Build history of the part. All positions in model axes, mm. A direction names the side the tool comes from. Give positions to 0.01 mm unless a question says otherwise; leave off trailing zeros. Loops run counter-clockwise (first coordinate to the right, second up) from the corner with the lowest first, then second, coordinate; pieces in that order, holes last.
1) Two-plate mould, pull along Z, no slides. Class faces 6 (the flat face through (28, 1, 23)), 7 (the flat face through (-22.4, 22, 12.4)), 8 (the flat face through (0, 12, 12)), 9 (the flat face through (-22, 12, 12)): +Z half, -Z half, draft (parallel to the pull), parting line (faces both ways), or undercut.
2) 3-axis set-ups, long thin cutter, end or side, ignore diameter. For faces 1 (the flat face through (16, 2, 12)), 2 (the flat face through (-10, 0, 12)), 3 (the flat face through (-23, 12, 12)), 4 (the flat face through (0, 12, 2)), 5 (the flat face through (-22, 12, 23)): which of +Z, -Z, +X, -X, +Y, -Y reach the whole face in a straight line?
3) Band-saw the part on C-C on x = 22. List the corners of the cut face in (y, z), then the cut area to 3 significant figures.
4) Flat gauge pins, fed straight in: P1, Ø10, axis at y = 8, z = 10, coming from the +X side; P2, Ø5, axis at y = 13, z = 3, coming from the -X side; P3, Ø12.5, axis at x = -30.5, z = 11, coming from the +Y side. Where does each tip first touch, or does it go through?
5) Wall check: line 1 (X direction, y = 15.5, z = 1.5); line 2 (Y direction, x = -29, z = 17.75); line 3 (X direction, y = 1.5, z = 6). Give the ranges that are in metal, low to high.
6) Band-saw the part on A-A on y = 13.25. List the corners of the cut face in (x, z), then the cut area to 3 significant figures.
7) Band-saw the part on B-B on z = 6.75. List the corners of the cut face in (x, y).
8) Band-saw the part on D-D on x = -14. List the corners of the cut face in (y, z).
```python
from build123d import *

# Parameters (mm, degrees)
F0_W     = 30
F0_H     = 2
F0_W_2   = 11
F0_H_2   = 1
F1_DEPTH = 25
F2_SIZE  = 5
F3_R     = 1
F7_SIZE  = 2


with BuildPart() as f1:
    # F0 (on Top) → F1 (new body)
    with BuildSketch(Plane.XY):
        with Locations((16, 1)):
            Rectangle(F0_W, F0_H)
        Polygon((0, 1), (0, 0), (1, 0), (1, 2), (1, 22), (0, 22), align=None)
        with Locations((-5.5, 0.5)):
            Rectangle(F0_W_2, F0_H_2)
    extrude(amount=F1_DEPTH)

    # F2
    f2_edges = [f1.edges().sort_by_distance(p)[0] for p in [
        (31, 1, 0),
        (31, 1, 25),
    ]]
    chamfer(f2_edges, length=F2_SIZE)

    # F3
    f3_edges = [f1.edges().sort_by_distance(p)[0] for p in [
        (0, 1, 12.5),
    ]]
    fillet(f3_edges, radius=F3_R)

    # F4 (on face) → F5 (join, up to the next surface of F1)
    with BuildSketch(Plane(origin=(0, 22, 0), x_dir=(-1, 0, 0), z_dir=(0, 1, 0))):
        with BuildLine():
            ThreePointArc((0.5, 5), (0.3535533906, 5.3535533906), (0, 5.5))
            Line((0, 5.5), (0, 4.5))
            ThreePointArc((0, 4.5), (0.3535533906, 4.6464466094), (0.5, 5))
        make_face()
        with BuildLine():
            ThreePointArc((0, 19.5), (0.3535533906, 19.6464466094), (0.5, 20))
            ThreePointArc((0.5, 20), (0.3535533906, 20.3535533906), (0, 20.5))
            Line((0, 20.5), (0, 19.5))
        make_face()
    extrude(until=Until.NEXT, dir=(0, -1, 0))

    # F6: F1 across face


with BuildPart() as f1_1:
    add(f1.part)
    add(f1.part.mirror(Plane(origin=(-11, 0.5, 12.5), x_dir=(0, -1, 0), z_dir=(-1, 0, 0))))

    # F7
    f7_edges = [f1_1.edges().sort_by_distance(p)[0] for p in [
        (-22.5, 22, 25),
        (-22.5, 22, 0),
        (0.5, 22, 25),
        (0.5, 22, 0),
    ]]
    chamfer(f7_edges, length=F7_SIZE)


solid = f1_1.part
```
Findings below:
1. face 6: +Z half
1. face 7: draft
1. face 8: undercut
1. face 9: undercut
2. face 1: +Z, -Z, +X, +Y
2. face 2: +Z, -Z, +X, -X, -Y
2. face 3: +Z, -Z, -X, +Y
2. face 4: -Z, +Y
2. face 5: +Z, +Y
3. outline: (0, 0) - (2, 0) - (2, 25) - (0, 25) - close
3. area: 50.0 mm2
4. P1: stops at x = 1
4. P2: stops at x = -23
4. P3: stops at y = 2
5. line 1: x = -23 to -22, 0 to 1
5. line 2: y = 0 to 2
5. line 3: x = -53 to -21.87, -0.13 to 31
6. outline: (-23, 0) - (-22, 0) - (-22, 4.5) arc R0.5 ccw to (-22, 5.5) - (-22, 19.5) arc R0.5 ccw to (-22, 20.5) - (-22, 25) - (-23, 25) - close; (0, 0) - (1, 0) - (1, 25) - (0, 25) - (0, 20.5) arc R0.5 ccw to (0, 19.5) - (0, 5.5) arc R0.5 ccw to (0, 4.5) - close
6. area: 51.6 mm2
7. outline: (-53, 0) - (31, 0) - (31, 2) - (1, 2) - (1, 22) - (0, 22) - (0, 2) arc R1 cw to (-1, 1) - (-21, 1) arc R1 cw to (-22, 2) - (-22, 22) - (-23, 22) - (-23, 2) - (-53, 2) - close
8. outline: (0, 0) - (1, 0) - (1, 25) - (0, 25) - close
